```python
from build123d import *

# Parameters (mm, degrees)
F0_R            = 115
F0_R_2          = 70
F1_DEPTH        = 5
F2_R            = 5
F3_DEPTH        = 25
F3_COPIES_COUNT = 12


# Not quite as in the source:
# - a pattern or mirror of a feature is missing from the dataset's text; its kind, count and spacing are read off the source's solid


with BuildPart() as f1:
    # F0 (on Top) → F1 (new body)
    with BuildSketch(Plane.XY):
        Circle(F0_R)
        Circle(F0_R_2, mode=Mode.SUBTRACT)
    extrude(amount=F1_DEPTH)

    # F2 (on face) → F3 (cut)
    with BuildSketch(Plane.XY.offset(5)):
        with Locations((0, 92.5)):
            Circle(F2_R)
    f3 = extrude(amount=-F3_DEPTH, mode=Mode.SUBTRACT)

    # F3_copies: F3 ×12 about axis
    f3_copies_axis = Axis((0, 0, 0), (0, 0, 1))
    for i in range(1, F3_COPIES_COUNT):
        add(f3.rotate(f3_copies_axis, i * 360 / F3_COPIES_COUNT), mode=Mode.SUBTRACT)


solid = f1.part
```
Design review of the part built by this model. Coordinates are the model's own, in mm. Give positions to 0.01 mm unless a question says otherwise; leave off trailing zeros. Write each loop counter-clockwise with the first axis right and the second up, starting at its lowest first coordinate (ties: lowest second). Pieces come first, ordered by that corner, then holes.
(1) Add section D-D (z = 3.45). Give the number of separate pieces and of enclosed holes in the cut face, and give its area (3 significant figures).
Checked values:
separate pieces: 1
enclosed holes: 13
area: 25,200 mm2
(2) Clearance check with flat-ended pins moving along their axes: pin 1 Ø3 at (x, z) = (-89.5, 4) entering from -Y; pin 2 Ø1.5 at (y, z) = (1, 0.5) entering from -X; pin 3 Ø1 at (x, z) = (23, 2) entering from +Y. State where each tip first meets the part, or that it passes through.
Checked values:
pin 1: stops at y = -74.03
pin 2: stops at x = -115
pin 3: stops at y = 112.78
(3) Add section C-C (y = -29.5). Give the boundary of the cut face in (x, z).
Checked values:
outline: (-111.15, 0) - (-63.48, 0) - (-63.48, 5) - (-111.15, 5) - close; (63.48, 0) - (111.15, 0) - (111.15, 5) - (63.48, 5) - close
(4) Wall thickness on line 1 along Y through (x, z) = (0, 2); line 2 along Y through (x, z) = (-80.5, 3.75); line 3 along X through (y, z) = (1, 0.4): over which ranges is each line inside the solid? List them lowest first.
Checked values:
line 1: y = -115 to -97.5, -87.5 to -70, 70 to 87.5, 97.5 to 115
line 2: y = -82.13 to -51.23, -41.27 to 41.27, 51.23 to 82.13
line 3: x = -115 to -97.4, -87.6 to -69.99, 69.99 to 87.6, 97.4 to 115
(5) Mouldability with a two-part tool opening along Y and no side actions: class faces 1 (the face through (50, -50, 5)), 2 (the face through (-1.08, 87.62, 2.54)), 3 (the face through (-24.93, -112.265, 2.465)) as +Y half, -Y half, draft (parallel to the pull), parting line (faces both ways), or undercut.
Checked values:
face 1: draft
face 2: undercut
face 3: parting line
(6) Add section A-A (y = 0). Give the boundary of the cut face in (x, z), and give its area (3 significant figures).
Checked values:
outline: (-115, 0) - (-97.5, 0) - (-97.5, 5) - (-115, 5) - close; (-87.5, 0) - (-70, 0) - (-70, 5) - (-87.5, 5) - close; (70, 0) - (87.5, 0) - (87.5, 5) - (70, 5) - close; (97.5, 0) - (115, 0) - (115, 5) - (97.5, 5) - close
area: 350 mm2
